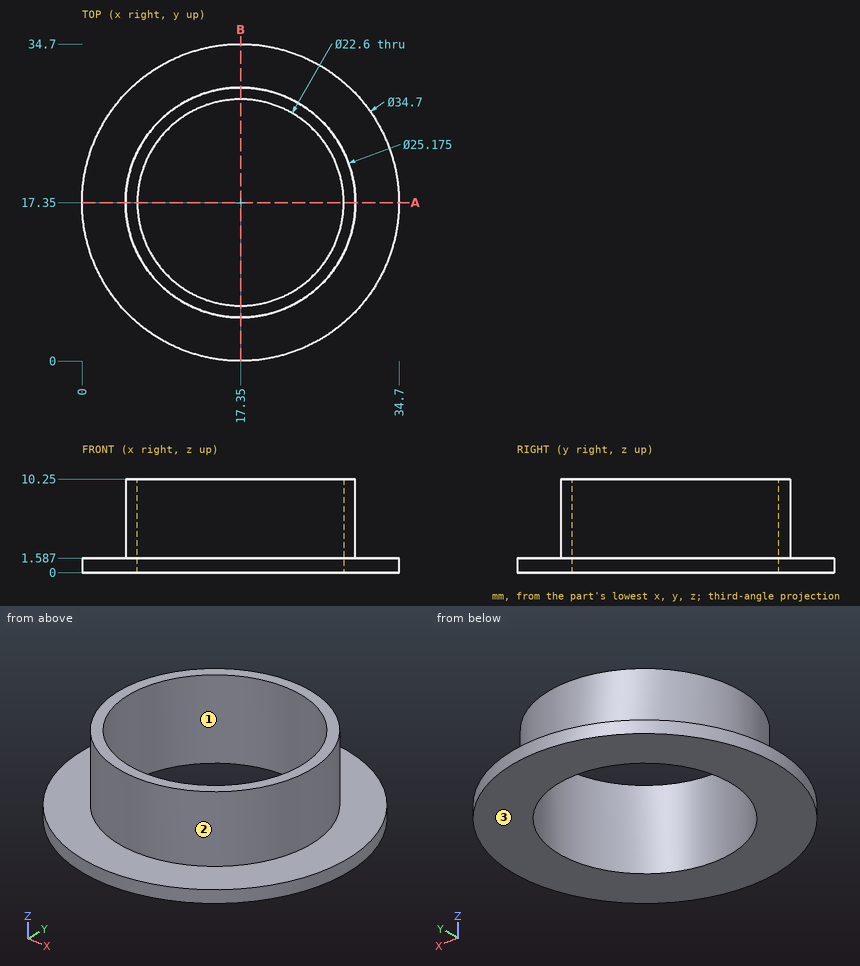
Design review of the part shown in the three views and the two pictorial views. Dimensions are in mm from the part's minimum x, y and z. Round coordinates to 2 decimals unless told otherwise and drop trailing zeros. Loops run counter-clockwise (first coordinate to the right, second up) from the corner with the lowest first, then second, coordinate; pieces in that order, holes last. Notation, with made-up numbers: M 78,87.25 L 127,87.25 A15 cw 127,102.25 Z; hole C 60.25,-14.5 d11. An arc over 180 degrees is marked long. Answer as a JSON object with one key per item and string values.
Item 1: The part is to be moulded in two halves that separate along Y. For the marked faces 1, 2 and 3, say which applies: pulls with the +Y half, pulls with the -Y half, needs draft (parallel to the pull), parting line crosses it, or undercut.
Answer sheet:
{"face 1": "undercut", "face 2": "parting line crosses it", "face 3": "needs draft"}
Item 2: We need section A-A on y = 17.35. Give the boundary of the cut face in (x, z).
Answer sheet:
{"outline": "M 0,0 L 6.05,0 L 6.05,10.25 L 4.76,10.25 L 4.76,1.59 L 0,1.59 Z; M 28.65,0 L 34.7,0 L 34.7,1.59 L 29.94,1.59 L 29.94,10.25 L 28.65,10.25 Z"}
Item 3: Clearance check with flat-ended pins moving along their axes: P1, Ø6, axis at x = 29.5, y = 29, coming from the -Z side; P2, Ø1.5, axis at x = 8.5, z = 3.5, coming from the +Y side (1 decimal); P3, Ø1, axis at x = 21, y = 4.5, coming from the +Z side; P4, Ø2, axis at x = 25.5, z = 6.5, coming from the -Y side. State where each tip first meets the part, or that it passes through.
Answer sheet:
{"P1": "stops at z = 0", "P2": "stops at y = 27", "P3": "stops at z = 1.59", "P4": "stops at y = 6.99"}
Item 4: Wall thickness on L1, parallel to Y at x = 17.35, z = 5.25; L2, parallel to Z at x = 7, y = 8.5; L3, parallel to Y at x = 26.5, z = 4.25 (1 decimal): over which ranges is each line inside the solid? List them lowest first. Write a range as from..to.
Answer sheet:
{"L1": "y = 4.76..6.05, 28.65..29.94", "L2": "z = 0..1.59", "L3": "y = 8.7..10.7, 24..26"}
